Autodesk Inventor part; units mm, degrees
ref_plane "YZ Plane" through (0, 0, 0) normal (1, 0, 0) x (0, 1, 0)
ref_plane "XZ Plane" through (0, 0, 0) normal (0, 1, 0) x (-1, 0, 0)
ref_plane "XY Plane" through (0, 0, 0) normal (0, 0, 1) x (1, 0, 0)
sketch "Sketch1" plane through (0, 0, 0) normal (0, 1, 0) x (-1, 0, 0)
  line L0 (-5, 50) -> (5, 50)
  line L1 (5, 50) -> (5, -50)
  line L2 (5, -50) -> (-5, -50)
  line L3 (-5, -50) -> (-5, 50)
  line L4 (-5, 50) -> (5, -50) construction
  line L5 (5, 50) -> (-5, -50) construction
  circle A0 centre (0, 45) radius 1.65
  circle A1 centre (0, -45) radius 1.65
  line L6 (0, 45) -> (0, -45) construction
  line L7 (-5, -10) -> (5, -10)
  line L8 (5, -10) -> (5, 10)
  line L9 (5, 10) -> (-5, 10)
  line L10 (-5, 10) -> (-5, -10)
  line L11 (-5, -10) -> (5, 10) construction
  line L12 (5, -10) -> (-5, 10) construction
  point P0 (0, 0)
  dimension "d0" = 90
  dimension "d1" = 5
  dimension "d2" = 3.3
  dimension "d3" = 10
  dimension "d4" = 20
extrude "Extrusion1" add sketch "Sketch1" along normal blind 5 contours L0 L1 L9 L3 | L7 L1 L2 L3
sketch "Sketch2" plane through (0, 5, 0) normal (0, 1, 0) x (1, 0, 0)
  line L0 (5, -50) -> (5, -10)
  line L1 (5, -10) -> (-5, -10)
  line L2 (-5, -10) -> (-5, -50)
  line L3 (-5, -50) -> (5, -50)
  circle A0 centre (0, -45) radius 1.65
  line L4 (-5, 50) -> (-5, 10)
  line L5 (-5, 10) -> (5, 10)
  line L6 (5, 10) -> (5, 50)
  line L7 (5, 50) -> (-5, 50)
  circle A1 centre (0, 45) radius 1.65
  line L8 (-5, -35) -> (5, -35)
  line L9 (5, -35) -> (5, 17)
  line L10 (5, 17) -> (-5, 17)
  line L11 (-5, 17) -> (-5, -35)
  point P0 (0, 0)
  point P1 (5, -35)
  point P2 (-5, 17)
  dimension "d7" = 52
  dimension "d26" = 7
extrude "Extrusion2" add sketch "Sketch2" along normal blind 5 contours L8 L2 L1 L0 | L1 L11 L5 L9 | L5 L4 L10 L6
sketch "Sketch3" plane through (0, 10, 0) normal (0, 1, 0) x (1, 0, 0)
  line L0 (5, -35) -> (5, 17)
  line L1 (5, 17) -> (-5, 17)
  line L2 (-5, 17) -> (-5, -35)
  line L3 (-5, -35) -> (5, -35)
  line L4 (-5, -5) -> (0, -5)
  line L5 (0, -5) -> (0, -35)
  line L6 (0, -35) -> (-5, -35)
  line L7 (-5, -35) -> (-5, -5)
  point P0 (0, 0)
  point P1 (-5, -35)
  point P2 (0, -35)
  dimension "d10" = 5
  dimension "d11" = 30
extrude "Extrusion3" add sketch "Sketch3" along normal blind 14 contours L3 L2 L4 L5
sketch "Sketch4" plane through (-5, 0, -50) normal (-1, 0, 0) x (0, 0, 1)
  line L0 (0, 0) -> (40, 0)
  line L1 (40, 0) -> (40, 5)
  line L2 (40, 5) -> (60, 5)
  line L3 (60, 0) -> (60, 5)
  line L4 (60, 0) -> (100, 0)
  line L5 (100, 0) -> (100, 5)
  line L6 (85, 5) -> (100, 5)
  line L7 (85, 5) -> (85, 24)
  line L8 (33, 10) -> (55, 10)
  line L9 (55, 24) -> (85, 24)
  line L10 (55, 10) -> (55, 24)
  line L11 (33, 5) -> (33, 10)
  line L12 (0, 5) -> (33, 5)
  line L13 (0, 0) -> (0, 5)
  line L14 (56, 6.1345) -> (84, 6.1345)
  line L15 (84, 6.1345) -> (84, 22.1345)
  line L16 (84, 22.1345) -> (56, 22.1345)
  line L17 (56, 22.1345) -> (56, 6.1345)
  circle A0 centre (59, 19.1345) radius 1.5
  circle A1 centre (81, 9.1345) radius 1.5
  line L18 (84, 6.1345) -> (81, 6.1345) construction
  line L19 (81, 6.1345) -> (81, 9.1345) construction
  line L20 (81, 9.1345) -> (84, 9.1345) construction
  line L21 (84, 9.1345) -> (84, 6.1345) construction
  line L22 (56, 22.1345) -> (59, 22.1345) construction
  line L23 (59, 22.1345) -> (59, 19.1345) construction
  line L24 (59, 19.1345) -> (56, 19.1345) construction
  line L25 (56, 19.1345) -> (56, 22.1345) construction
  point P0 (50, 0)
  point P1 (70, 22.1345)
  point P2 (70, 24)
  dimension "d14" = 28
  dimension "d15" = 16
  dimension "d18" = 3
  dimension "d19" = 3
  dimension "d22" = 3
  dimension "d23" = 3
  dimension "d24" = 3
  dimension "d25" = 3
extrude "Extrusion4" cut sketch "Sketch4" against normal through all contours A0 | A1
sketch "Sketch5" plane through (0, 5, 0) normal (0, 1, 0) x (1, 0, 0)
  circle A0 centre (0, 45) radius 1.65
  line L0 (5, -35) -> (-5, -35)
  line L1 (-5, -35) -> (-5, -50)
  line L2 (-5, -50) -> (5, -50)
  line L3 (5, -50) -> (5, -35)
  circle A1 centre (0, -45) radius 1.65
  line L4 (-5, 17) -> (5, 17)
  line L5 (5, 17) -> (5, 50)
  line L6 (5, 50) -> (-5, 50)
  line L7 (-5, 50) -> (-5, 17)
  circle A2 centre (0, 45) radius 1.65
  circle A3 centre (0, 45) radius 2.9
  circle A4 centre (0, -45) radius 2.9
  point P0 (0, 0)
  dimension "d27" = 5.8
  dimension "d28" = 5.8
extrude "Extrusion5" cut sketch "Sketch5" against normal blind 3.3 contours A0 | A1 | A3 | A4
chamfer "Chamfer1" distance 4 angle 45 2 edges at (0, 5, 35) (-2.5, 10, 5)
fillet "Fillet1" radius 2 2 edges at (-2.5, 24, 35) (-2.5, 24, 5)
sketch "Sketch6" plane through (5, 0, 50) normal (1, 0, 0) x (0, 0, -1)
  arc A0 (17.7749, 10) -> (20.2251, 10) centre (19, 9.1345) ccw
  line L0 (15, 10) -> (17.7749, 10)
  line L1 (15, 9) -> (15, 10)
  line L2 (11, 5) -> (15, 9)
  line L3 (0, 5) -> (11, 5)
  line L4 (0, 0) -> (0, 5)
  line L5 (0, 0) -> (40, 0)
  line L6 (40, 0) -> (40, 5)
  line L7 (40, 5) -> (60, 5)
  line L8 (60, 0) -> (60, 5)
  line L9 (60, 0) -> (100, 0)
  line L10 (100, 0) -> (100, 5)
  line L11 (67, 5) -> (100, 5)
  line L12 (67, 5) -> (67, 10)
  line L13 (20.2251, 10) -> (67, 10)
  circle A1 centre (19, 9.1345) radius 2.9
  point P0 (50, 0)
  dimension "d35" = 5.8
extrude "Extrusion6" cut sketch "Sketch6" against normal up to surface (5 mm away) contours L0 A1 L13 A0 | A0 L13 A1 L0
chamfer "Chamfer2" distance 5 angle 45 1 edges at (0, 5, -17)
fillet "Fillet2" radius 2 4 edges at (-5, 2.5, 50) (5, 2.5, 50) (-5, 2.5, -50) (5, 2.5, -50)
properties part number "SOPORTE_FIN_CARRERA_INGRESO" material "Steel, Mild, Welded"
Check sheet for the modelled part. Datum: model origin and axes. Units: mm. A direction names the side the tool comes from. Coordinates: 2 decimals unless noted, no trailing zeros. Loops run counter-clockwise (first coordinate to the right, second up) from the corner with the lowest first, then second, coordinate; pieces in that order, holes last. Notation, with made-up numbers: (14.5, 58) -> (24.5, 58) arc R10 cw to (24.5, 68) -> close; hole circle Ø9 at (27, 55). An arc over 180 degrees is marked (long way). Answer in a Markdown table with one row per item.
1. Sectioned sample at D-D, the plane z = -45. Record the boundary of the cut face in (x, y), then the cut area to 4 significant figures.
Check values:
| item | result |
|---|---|
| outline | (-5, 0) -> (-1.65, 0) -> (-1.65, 1.7) -> (-2.9, 1.7) -> (-2.9, 5) -> (-5, 5) -> close; (1.65, 0) -> (5, 0) -> (5, 5) -> (2.9, 5) -> (2.9, 1.7) -> (1.65, 1.7) -> close |
| area | 25.25 mm2 |
2. Sectioned sample at C-C, the plane z = 19. Record the boundary of the cut face in (x, y).
Check values:
| item | result |
|---|---|
| outline | (-5, 0) -> (5, 0) -> (5, 10) -> (0, 10) -> (0, 24) -> (-5, 24) -> close |
3. Access from +Z, -Z, +X, -X, +Y, -Y to the whole of each face (thin tool, end or side, straight path). Record for faces 1 (the face through (0, 2, 10)), 2 (the face through (-0.63, 3.37, -42.17)), 3 (the face through (0, 5, -36)), 4 (the face through (1, 10, 0)).
Check values:
| item | result |
|---|---|
| face 1 | +X, -X, -Y |
| face 2 | +Y |
| face 3 | -Z, +X, -X, +Y |
| face 4 | -Z, +X, +Y |
4. Release check for a two-part mould opening along X. For faces 5 (the face through (-2.46, 23.4, 5.57)), 6 (the face through (-4.43, 2.54, 49.4)), 7 (the face through (0.215, 0.838, -46.636)), 8 (the face through (2, 1.7, 45)) record: released by +X, released by -X, zero draft, split by the parting line, or undercut.
Check values:
| item | result |
|---|---|
| face 5 | zero draft |
| face 6 | released by -X |
| face 7 | undercut |
| face 8 | undercut |
5. Material ranges on line 1 along Z through (x, y) = (0, 1.3); line 2 along Z through (x, y) = (0, 3.65); line 3 along X through (y, z) = (2.75, -45), recorded low to high. Write a range as [from, to].
Check values:
| item | result |
|---|---|
| line 1 | z = [-50, -46.65], [-43.35, -10], [10, 43.35], [46.65, 50] |
| line 2 | z = [-50, -47.9], [-42.1, -10], [10, 42.1], [47.9, 50] |
| line 3 | x = [-5, -2.9], [2.9, 5] |
6. Go/stop test with flat-tipped pins: pin 1 (2 mm diameter, centred on x = 3.5, y = 9, fed in from +Z); pin 2 (5 mm diameter, centred on x = 2, z = 1, fed in from -Y); pin 3 (1.7 mm diameter, centred on x = -0.5, z = 46.5, fed in from +Y). Record where each tip stops, or that it passes through.
Check values:
| item | result |
|---|---|
| pin 1 | stops at z = 36 |
| pin 2 | stops at y = 5 |
| pin 3 | stops at y = 1.7 |
7. Sectioned sample at A-A, the plane z = 9. Record the boundary of the cut face in (x, y).
Check values:
| item | result |
|---|---|
| outline | (-5, 5) -> (5, 5) -> (5, 10) -> (0, 10) -> (0, 17.63) -> (-5, 17.63) -> close; (-5, 20.63) -> (0, 20.63) -> (0, 24) -> (-5, 24) -> close |
8. Sectioned sample at B-B, the plane z = 31. Record the boundary of the cut face in (x, y), then the cut area to 3 significant figures.
Check values:
| item | result |
|---|---|
| outline | (-5, 0) -> (5, 0) -> (5, 6.23) -> (0, 6.23) -> (0, 7.63) -> (-5, 7.63) -> close; (-5, 10.63) -> (0, 10.63) -> (0, 24) -> (-5, 24) -> close |
| area | 136 mm2 |
